from build123d import *

# Parameters (mm, degrees)
SKETCH1_W                = 73
SKETCH1_H                = 35
BOSS_EXTRUDE1_DEPTH      = 5
SKETCH2_W                = 92
SKETCH2_H                = 35
BOSS_EXTRUDE2_DEPTH      = 3
M3_CLEARANCE_HOLE1_D     = 4
M3_CLEARANCE_HOLE1_DEPTH = 10
M3_CLEARANCE_HOLE1_TIP   = 1.201721238
SKETCH9_W                = 73
SKETCH9_H                = 8
BOSS_EXTRUDE3_DEPTH      = 20
M3_CLEARANCE_HOLE3_D     = 3.6
M3_CLEARANCE_HOLE3_DEPTH = 10
M3_CLEARANCE_HOLE3_TIP   = 1.081549114
SKETCH12_W               = 53
SKETCH12_H               = 35
CUT_EXTRUDE1_DEPTH       = 9
CHAMFER1_SIZE            = 10


with BuildPart() as part:
    # Sketch1 → Boss-Extrude1 (new body)
    with BuildSketch(Plane(origin=(0, 0, 0), x_dir=(1, 0, 0), z_dir=(0, 1, 0))):
        Rectangle(SKETCH1_W, SKETCH1_H)
    extrude(amount=BOSS_EXTRUDE1_DEPTH)

    # Sketch2 → Boss-Extrude2 (add)
    with BuildSketch(Plane.XZ):
        Rectangle(SKETCH2_W, SKETCH2_H)
    extrude(amount=BOSS_EXTRUDE2_DEPTH)

    # M3 Clearance Hole1
    with Locations(Plane(origin=(0, 0, 0), x_dir=(1, 0, 0), z_dir=(0, 1, 0))):
        with Locations((-41, 12.5), (-41, -12.5), (41, 12.5), (41, -12.5)):
            Hole(M3_CLEARANCE_HOLE1_D / 2, depth=M3_CLEARANCE_HOLE1_DEPTH)
            with Locations((0, 0, -(M3_CLEARANCE_HOLE1_DEPTH + M3_CLEARANCE_HOLE1_TIP / 2))):  # 118° drill point
                Cone(0, M3_CLEARANCE_HOLE1_D / 2, M3_CLEARANCE_HOLE1_TIP, mode=Mode.SUBTRACT)

    # Sketch9 → Boss-Extrude3 (add)
    with BuildSketch(Plane(origin=(0, 0, -17.5), x_dir=(-1, 0, 0), z_dir=(0, 0, -1))):
        with Locations((0, 1)):
            Rectangle(SKETCH9_W, SKETCH9_H)
    extrude(amount=BOSS_EXTRUDE3_DEPTH)

    # M3 Clearance Hole3
    with Locations(Plane(origin=(0, 5, 0), x_dir=(1, 0, 0), z_dir=(0, 1, 0))):
        with Locations((-20.6, -12.5), (-19.3, 33.1), (31.5, -10), (31.5, 17.9)):
            Hole(M3_CLEARANCE_HOLE3_D / 2, depth=M3_CLEARANCE_HOLE3_DEPTH)
            with Locations((0, 0, -(M3_CLEARANCE_HOLE3_DEPTH + M3_CLEARANCE_HOLE3_TIP / 2))):  # 118° drill point
                Cone(0, M3_CLEARANCE_HOLE3_D / 2, M3_CLEARANCE_HOLE3_TIP, mode=Mode.SUBTRACT)

    # Sketch12 → Cut-Extrude1 (cut, through all)
    with BuildSketch(Plane(origin=(0, 5, 0), x_dir=(1, 0, 0), z_dir=(0, 1, 0))):
        with Locations((0, 10)):
            Rectangle(SKETCH12_W, SKETCH12_H)
    extrude(amount=-CUT_EXTRUDE1_DEPTH, mode=Mode.SUBTRACT)

    # Chamfer1
    chamfer1_edges = [part.edges().sort_by_distance(p)[0] for p in [
        (36.5, 1, -37.5),
        (-36.5, 1, -37.5),
    ]]
    chamfer(chamfer1_edges, length=CHAMFER1_SIZE)


solid = part.part
The listing builds one solid part. Answer for the finished solid, in the listing's coordinates (mm). A direction names the side the tool comes from. Coordinates: 2 decimals unless noted, no trailing zeros. Loops run counter-clockwise (first coordinate to the right, second up) from the corner with the lowest first, then second, coordinate; pieces in that order, holes last.
1) Find section A-A on z = -22.5. Write down the section's boundary in (x, y).
2) Flat-ended cylindrical pins translate along their axes: pin 1 Ø1.5 at (x, y) = (-42, -2) entering from -Z; pin 2 Ø5 at (x, z) = (-41.5, 8) entering from +Y; pin 3 Ø4 at (y, z) = (4, 6) entering from -X. Find the tip coordinate at first contact, or state that the pin passes through.
3) Find section D-D on x = 8.5. Write down the section's boundary in (y, z).
4) Find section C-C on y = 2.5. Write down the section's boundary in (x, z).
5) Find section B-B on x = 31.5. Write down the section's boundary in (y, z), then the cut area to 3 significant figures.
6) Determine the mould class of faces 5 (the face through (-1, 1, 17.5)), 6 (the face through (-26.5, 1, -10)), 7 (the face through (41, 0, 0)), 8 (the face through (0, 1, -27.5)) for opening direction Z: pulls with the +Z half, pulls with the -Z half, needs draft (parallel to the pull), parting line crosses it, or undercut.
7) Find the intervals of material crossed by L1, parallel to X at y = -1.7, z = 12.5; L2, parallel to X at y = -1.8, z = -12.5; L3, parallel to X at y = -1.25, z = -17.9, in increasing order.
8) A tool of negligible diameter and unlimited length cuts with its end or side. For faces 1 (the face through (41, -1, -17.5)), 2 (the face through (-41, 0, 0)), 3 (the face through (1, -3, 9)), 4 (the face through (0, 1, 7.5)), from which of +Z, -Z, +X, -X, +Y, -Y can it reach the whole face along a straight path? Write none if from no direction.
Values:
1. outline: (-36.5, -3) - (-26.5, -3) - (-26.5, 5) - (-36.5, 5) - close; (26.5, -3) - (36.5, -3) - (36.5, 5) - (26.5, 5) - close
2. pin 1: stops at z = -17.5
2. pin 2: stops at y = 0
2. pin 3: stops at x = -36.5
3. outline: (-3, -37.5) - (5, -37.5) - (5, -27.5) - (-3, -27.5) - close; (-3, 7.5) - (5, 7.5) - (5, 17.5) - (-3, 17.5) - close
4. outline: (-36.5, -27.5) - (-26.5, -37.5) - (26.5, -37.5) - (36.5, -27.5) - (36.5, 17.5) - (-36.5, 17.5) - close; hole (-26.5, -27.5) - (26.5, -27.5) - (26.5, 7.5) - (-26.5, 7.5) - close; hole circle Ø3.6 at (-20.6, 12.5); hole circle Ø3.6 at (-19.3, -33.1); hole circle Ø3.6 at (31.5, -17.9); hole circle Ø3.6 at (31.5, 10)
5. outline: (-3, -32.5) - (5, -32.5) - (5, -19.7) - (-3, -19.7) - close; (-3, -16.1) - (5, -16.1) - (5, 8.2) - (-3, 8.2) - close; (-3, 11.8) - (5, 11.8) - (5, 17.5) - (-3, 17.5) - close
5. area: 342 mm2
6. face 5: pulls with the +Z half
6. face 6: undercut
6. face 7: needs draft
6. face 8: undercut
7. L1: x = -46 to -43, -39 to -22.4, -18.8 to 39, 43 to 46
7. L2: x = -46 to -43, -39 to -26.5, 26.5 to 39, 43 to 46
7. L3: x = -36.5 to -26.5, 26.5 to 29.7, 33.3 to 36.5
8. face 1: -Z, +X, +Y, -Y
8. face 2: +Z, -Z, -X, +Y
8. face 3: +Z, -Z, +X, -X, -Y
8. face 4: +Y, -Y
